Read the model definition and answer for the solid it produces. Units are mm, in the model's axes. Face numbers are marked on the shaded views. Round coordinates to 2 decimals unless told otherwise and drop trailing zeros. Order: outer loops, then holes, each group sorted by start corner. A loop starts at its lowest first (then second) coordinate and runs counter-clockwise, first axis right, second up. Notation, with made-up numbers: (-32.5, -10) -> (-21.5, -10) arc R12 cw to (-21.5, 2) -> close; hole circle Ø8 at (43.25, 29). An arc over 180 degrees is marked (long way). One line per item, written item: value. Start each with the question number.
1. Section C-C (z = -54) is taken. Give the vertices of the cut face in (x, y), then the cut area to 3 significant figures.
2. The mould has two halves that part along X. Classify the marked faces 1 and 2: released by +X, released by -X, zero draft, split by the parting line, or undercut.
3. A flat-ended cylindrical pin translates along its axis: pin 1 Ø0.9 at (x, z) = (2, 42) entering from +Y. Find the tip coordinate at first contact, or state that the pin passes through.
4. Consider line 1 (Y direction, x = 0.75, z = -45.5); line 2 (Y direction, x = 1.3, z = -13); line 3 (Z direction, x = 2.6, y = 36.5). Determine where each line is inside the solid, lowest interval first.
5. Section A-A (y = 60) is taken. Give the vertices of the cut face in (x, z), then the cut area to 3 significant figures.
6. Section B-B (x = 1.3) is taken. State how many separate pieces and enclosed holes the cut face has, then the cut area to 3 significant figures.
from build123d import *

# Parameters (mm, degrees)
SKETCH1_R           = 1.5
SKETCH1_R_2         = 2
BOSS_EXTRUDE1_DEPTH = 3
FILLET1_R           = 5
FILLET2_R           = 10
FILLET3_R           = 2
FILLET4_R           = 5
FILLET5_R           = 2
FILLET6_R           = 5
FILLET7_R           = 15
FILLET8_R           = 15
FILLET9_R           = 30
FILLET10_R          = 5
BOSS_EXTRUDE2_DEPTH = 3
CUT_EXTRUDE1_DEPTH  = 3


with BuildPart() as part:
    # Sketch1 → Boss-Extrude1 (new body)
    with BuildSketch(Plane(origin=(0, 0, 0), x_dir=(0, 0, -1), z_dir=(1, 0, 0))):
        with BuildLine():
            Line((-42.5, 0), (42.5, 0))
            ThreePointArc((42.5, 0), (48, 5.5), (42.5, 11))
            Line((42.5, 11), (41.335123714, 11))
            ThreePointArc((41.335123714, 11), (31.5, 18.546755856), (36.244089058, 30))
            Line((36.244089058, 30), (62.224851171, 45))
            Line((62.224851171, 45), (81.543367697, 50.176380902))
            Line((81.543367697, 50.176380902), (101.467261659, 48.433266047))
            Line((101.467261659, 48.433266047), (109.012004109, 72.000867593))
            Line((109.012004109, 72.000867593), (85.376618037, 67.833311329))
            Line((85.376618037, 67.833311329), (60, 56))
            Line((60, 56), (-60, 56))
            Line((-60, 56), (-85.376618037, 67.833311329))
            Line((-85.376618037, 67.833311329), (-109.012004109, 72.000867593))
            Line((-109.012004109, 72.000867593), (-101.467261659, 48.433266047))
            Line((-101.467261659, 48.433266047), (-81.543367697, 50.176380902))
            Line((-81.543367697, 50.176380902), (-62.224851171, 45))
            Line((-62.224851171, 45), (-36.244089058, 30))
            ThreePointArc((-36.244089058, 30), (-31.5, 18.546755856), (-41.335123714, 11))
            Line((-41.335123714, 11), (-42.5, 11))
            ThreePointArc((-42.5, 11), (-48, 5.5), (-42.5, 0))
        make_face()
        with Locations((31.5, 53.5)):
            Circle(SKETCH1_R, mode=Mode.SUBTRACT)
        with Locations((45.5, 42.5)):
            Circle(SKETCH1_R, mode=Mode.SUBTRACT)
        with Locations((70, 53.5)):
            Circle(SKETCH1_R_2, mode=Mode.SUBTRACT)
        with Locations((90.5, 64.384076231)):
            Circle(SKETCH1_R, mode=Mode.SUBTRACT)
        with Locations((102.5, 66.5)):
            Circle(SKETCH1_R, mode=Mode.SUBTRACT)
        with Locations((96.5, 52.5)):
            Circle(SKETCH1_R, mode=Mode.SUBTRACT)
        with Locations((42.5, 4.5)):
            Circle(SKETCH1_R, mode=Mode.SUBTRACT)
        with Locations((36.5, 4.5)):
            Circle(SKETCH1_R, mode=Mode.SUBTRACT)
        with Locations((19, 7.5)):
            Circle(SKETCH1_R, mode=Mode.SUBTRACT)
        with Locations((-36.5, 4.5)):
            Circle(SKETCH1_R, mode=Mode.SUBTRACT)
        with Locations((-42.5, 4.5)):
            Circle(SKETCH1_R, mode=Mode.SUBTRACT)
        with Locations((-96.5, 52.5)):
            Circle(SKETCH1_R, mode=Mode.SUBTRACT)
        with Locations((-102.5, 66.5)):
            Circle(SKETCH1_R, mode=Mode.SUBTRACT)
        with Locations((-90.5, 64.384076231)):
            Circle(SKETCH1_R, mode=Mode.SUBTRACT)
        with Locations((-70, 53.5)):
            Circle(SKETCH1_R_2, mode=Mode.SUBTRACT)
        with Locations((-45.5, 42.5)):
            Circle(SKETCH1_R, mode=Mode.SUBTRACT)
        with Locations((-31.5, 53.5)):
            Circle(SKETCH1_R, mode=Mode.SUBTRACT)
        with Locations((-19, 7.5)):
            Circle(SKETCH1_R, mode=Mode.SUBTRACT)
        with BuildLine():
            Line((18.022110342, 29.115638387), (1.25, 33.310573815))
            Line((1.25, 33.310573815), (1.25, 47))
            Line((1.25, 47), (26.25, 47))
            Line((26.25, 47), (34.109043647, 42.61417819))
            Line((34.109043647, 42.61417819), (33.125793941, 41.789133724))
            ThreePointArc((33.125793941, 41.789133724), (27.076764403, 38.174520246), (22.46666207, 32.845060102))
            Line((22.46666207, 32.845060102), (18.022110342, 29.115638387))
        make_face(mode=Mode.SUBTRACT)
        with BuildLine():
            Line((-18.022110342, 29.115638387), (-22.46666207, 32.845060102))
            ThreePointArc((-22.46666207, 32.845060102), (-27.076764403, 38.174520246), (-33.125793941, 41.789133724))
            Line((-33.125793941, 41.789133724), (-34.109043647, 42.61417819))
            Line((-34.109043647, 42.61417819), (-26.25, 47))
            Line((-26.25, 47), (-1.25, 47))
            Line((-1.25, 47), (-1.25, 33.310573815))
            Line((-1.25, 33.310573815), (-18.022110342, 29.115638387))
        make_face(mode=Mode.SUBTRACT)
        with BuildLine():
            Line((-13.030075377, 8.1), (13.030075377, 8.1))
            ThreePointArc((13.030075377, 8.1), (15.257332965, 12.189610161), (19.739088719, 13.454304986))
            ThreePointArc((19.739088719, 13.454304986), (18.820952742, 18.98346387), (19.311633684, 24.566814463))
            Line((19.311633684, 24.566814463), (0, 29.3969196))
            Line((0, 29.3969196), (-19.311633684, 24.566814463))
            ThreePointArc((-19.311633684, 24.566814463), (-18.820952742, 18.98346387), (-19.739088719, 13.454304986))
            ThreePointArc((-19.739088719, 13.454304986), (-15.257332965, 12.189610161), (-13.030075377, 8.1))
        make_face(mode=Mode.SUBTRACT)
    extrude(amount=BOSS_EXTRUDE1_DEPTH)

    # Fillet1
    fillet1_edges = [part.edges().sort_by_distance(p)[0] for p in [
        (1.5, 29.115638387, 18.022110342),
        (1.5, 32.845060102, 22.46666207),
    ]]
    fillet(fillet1_edges, radius=FILLET1_R)

    # Fillet2
    fillet2_edges = [part.edges().sort_by_distance(p)[0] for p in [
        (1.5, 29.3969196, 0),
    ]]
    fillet(fillet2_edges, radius=FILLET2_R)

    # Fillet3
    fillet3_edges = [part.edges().sort_by_distance(p)[0] for p in [
        (1.5, 8.1, -13.030075377),
        (1.5, 13.454304986, -19.739088719),
        (1.5, 24.566814463, -19.311633684),
        (1.5, 24.566814463, 19.311633684),
        (1.5, 13.454304986, 19.739088719),
        (1.5, 8.1, 13.030075377),
    ]]
    fillet(fillet3_edges, radius=FILLET3_R)

    # Fillet4
    fillet4_edges = [part.edges().sort_by_distance(p)[0] for p in [
        (1.5, 33.310573815, 1.25),
    ]]
    fillet(fillet4_edges, radius=FILLET4_R)

    # Fillet5
    fillet5_edges = [part.edges().sort_by_distance(p)[0] for p in [
        (1.5, 47, 1.25),
    ]]
    fillet(fillet5_edges, radius=FILLET5_R)

    # Fillet6
    fillet6_edges = [part.edges().sort_by_distance(p)[0] for p in [
        (1.5, 47, 26.25),
    ]]
    fillet(fillet6_edges, radius=FILLET6_R)

    # Fillet7
    fillet7_edges = [part.edges().sort_by_distance(p)[0] for p in [
        (1.5, 45, 62.224851171),
    ]]
    fillet(fillet7_edges, radius=FILLET7_R)

    # Fillet8
    fillet8_edges = [part.edges().sort_by_distance(p)[0] for p in [
        (1.5, 50.176380902, 81.543367697),
        (1.5, 56, 60),
    ]]
    fillet(fillet8_edges, radius=FILLET8_R)

    # Fillet9
    fillet9_edges = [part.edges().sort_by_distance(p)[0] for p in [
        (1.5, 67.833311329, 85.376618037),
    ]]
    fillet(fillet9_edges, radius=FILLET9_R)

    # Fillet10
    fillet10_edges = [part.edges().sort_by_distance(p)[0] for p in [
        (1.5, 48.433266047, 101.467261659),
        (1.5, 72.000867593, 109.012004109),
    ]]
    fillet(fillet10_edges, radius=FILLET10_R)

    # Sketch2 → Boss-Extrude2 (add)
    with BuildSketch(Plane.ZY):
        Polygon((34.109043647, 42.61417819), (31.155122873, 40.890234672), (35.435126155, 42.486892898), align=None)
    extrude(amount=-BOSS_EXTRUDE2_DEPTH)

    # Fillet11
    # an asymmetric fillet: 2, 1 mm, written as the material it adds along each edge
    with BuildSketch(Plane(origin=(0, 42.61417819, 34.109043647), x_dir=(0, 0.4873135344398375, -0.8732270719301786), z_dir=(1, 0, 0))) as fillet11_piece_1:
        with BuildLine():
            Bezier((2.913430357, 0), (0, 0), (1.191368957, -2.01710596), weights=[1, 0.495705063, 1])
            Line((1.191368957, -2.01710596), (0, 0))
            Line((0, 0), (2.913430357, 0))
        make_face()
    extrude(amount=3)

    # Sketch3 → Cut-Extrude1 (cut)
    with BuildSketch(Plane.ZY):
        Polygon((0, 0), (0, 75.071953776), (-134.912211469, 75.071953776), (-134.912211469, -12.246363453), align=None)
    extrude(amount=-CUT_EXTRUDE1_DEPTH, mode=Mode.SUBTRACT)

    # Mirror3: part across plane


with BuildPart() as part_1:
    add(part.part)
    add(part.part.mirror(Plane.XY))


solid = part_1.part
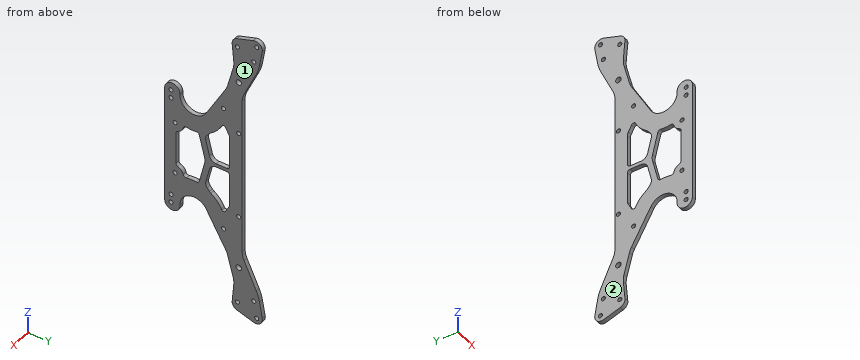
Answer:
1. outline: (0, 40.25) -> (3, 40.25) -> (3, 56) -> (0, 56) -> close
1. area: 47.2 mm^2
2. face 1: released by +X
2. face 2: released by -X
3. pin 1: y = 56
4. line 1: 0.89 to 10.11, 35.34 to 41, 44 to 56
4. line 2: 0 to 8.86, 26.15 to 30.37, 47 to 56
4. line 3: -47.5 to -25.29, -1.3 to 1.3, 25.29 to 47.5
5. outline: (0, -105.17) -> (3, -105.17) -> (3, -68.58) -> (0, -68.58) -> close; (0, 68.58) -> (3, 68.58) -> (3, 105.17) -> (0, 105.17) -> close
5. area: 220 mm^2
6. separate pieces: 1
6. enclosed holes: 21
6. area: 4,960 mm^2
